Model file for the job. Use its own axes, mm. A direction names the side the tool comes from. Coordinates: 2 decimals unless noted, no trailing zeros. Write each loop counter-clockwise with the first axis right and the second up, starting at its lowest first coordinate (ties: lowest second). Pieces come first, ordered by that corner, then holes. Notation, with made-up numbers: (-31, 12.25) -> (14, 12.25) arc R16 ccw to (14, 17.25) -> close; hole circle Ø5 at (50.25, -25.75). An arc over 180 degrees is marked (long way). Write item = value, one per line. Start each with the question number.
from build123d import *


with BuildPart() as part:
    # Sketch1 → Revolve1 (revolve)
    with BuildSketch(Plane.XY, mode=Mode.PRIVATE) as revolve1_sk:
        with BuildLine():
            Line((-2.3453217, 5.55498), (-0.63265685, 6.35))
            Line((-0.63265685, 6.35), (1.353716934, 6.35))
            Line((1.353716934, 6.35), (2.983459057, 5.396470607))
            ThreePointArc((2.983459057, 5.396470607), (3.06874832, 5.396101014), (3.1115, 5.4699027))
            Line((3.1115, 5.4699027), (3.1115, 7.065518))
            Line((3.1115, 7.065518), (2.325457711, 7.525415561))
            ThreePointArc((2.325457711, 7.525415561), (2.119870759, 7.73279205), (2.0447, 8.01496285))
            Line((2.0447, 8.01496285), (2.0447, 9.757918))
            ThreePointArc((2.0447, 9.757918), (1.878576238, 10.158976238), (1.477518, 10.3251))
            Line((1.477518, 10.3251), (-2.7428317, 10.3251))
            Line((-2.7428317, 10.3251), (-3.1115, 9.9564317))
            Line((-3.1115, 9.9564317), (-3.1115, 9.013317))
            Line((-3.1115, 9.013317), (-0.866916035, 8.616817304))
            ThreePointArc((-0.866916035, 8.616817304), (-0.63265685, 8.33755), (-0.866916035, 8.058282696))
            Line((-0.866916035, 8.058282696), (-2.7428317, 7.72690726))
            Line((-2.7428317, 7.72690726), (-2.7428317, 5.95249))
            Line((-2.7428317, 5.95249), (-2.3453217, 5.55498))
        make_face()
    revolve(revolve1_sk.sketch.rotate(Axis((-3.1115, 0, 0), (1, 0, 0)), 270), axis=Axis((-3.1115, 0, 0), (1, 0, 0)))


solid = part.part
(1) Saw through at C-C (x = -2). Give the cut face in (y, z).
(2) 3-axis set-ups, long thin cutter, end or side, ignore diameter. For faces 4 (the face through (-2.743, -5, -4)), 5 (the face through (2.045, 3.7, -7.3)), 6 (the face through (3.112, -4, 4)): which of +Z, -Z, +X, -X, +Y, -Y reach the whole face in a straight line?
(3) Drill centre lines: line 1 along Y through (x, z) = (-1, -1); line 2 along Y through (x, z) = (-2.5, 3.25); line 3 along Y through (x, z) = (0.05, 0). Where is each one in solid material? Low to high.
(4) Mould opens along Z. For faces 1 (the face through (-0.66, -3.95, -9.54)), 2 (the face through (0.37, -3.86, 5.04)), 3 (the face through (-3.112, 9, 2)) say: released by +Z, released by -Z, zero draft, split by the parting line, or undercut.
(5) Saw through at D-D (x = 1.75). Give the cut face in (y, z), then the cut area to 3 significant figures.
(6) Drop flat-ended pins along their axis: pin 1 Ø10 at (y, z) = (-3.5, 2.5) entering from +X; pin 2 Ø1 at (y, z) = (0.5, -6) entering from -X. Give the stop position or say it passes through.
Returned:
q1.outline = circle Ø20.65 at (0, 0); circle Ø15.72 at (0, 0); hole circle Ø17.63 at (0, 0); hole circle Ø11.43 at (0, 0)
q2.face_4 = -X
q2.face_5 = +X
q2.face_6 = +Z, -Z, +X, +Y, -Y
q3.line_1 = -10.28 to -8.58, -7.97 to -6.1, 6.1 to 7.97, 8.58 to 10.28
q3.line_2 = -9.8 to -8.29, -7.06 to -4.69, 4.69 to 7.06, 8.29 to 9.8
q3.line_3 = -10.33 to -6.35, 6.35 to 10.33
q4.face_1 = split by the parting line
q4.face_2 = undercut
q4.face_3 = zero draft
q5.outline = circle Ø20.51 at (0, 0); hole circle Ø12.24 at (0, 0)
q5.area = 213 mm2
q6.pin_1 = 3.11
q6.pin_2 = -2.74
